from build123d import *

# Parameters (mm, degrees)
SKETCH_1_W           = 200
SKETCH_1_H           = 213
EXTRUDE_1_DEPTH      = 4
EXTRUDE_2_DEPTH      = 54
CUT_EXTRUDE_2_DEPTH  = 298.880848663
CUT_EXTRUDE_3_DEPTH  = 42
SKETCH_7_R           = 1.8
SKETCH_7_R_2         = 11.5
CUT_EXTRUDE_4_DEPTH  = 282.53330176
MIRROR_START         = 176
MIRROR_1_OUTLINE_R   = 1.8
MIRROR_1_OUTLINE_R_2 = 11.5
MIRROR_1_DEPTH       = 3.5
SKETCH_8_W           = 27
SKETCH_8_H           = 28
CUT_EXTRUDE_5_DEPTH  = 6
SKETCH_9_W           = 27
SKETCH_9_H           = 20
CUT_EXTRUDE_6_DEPTH  = 21
CUT_EXTRUDE_START    = -54
CUT_EXTRUDE_7_DEPTH  = 54
SKETCH_12_R          = 2
EXTRUDE_3_DEPTH      = 10
SKETCH_14_W          = 21
SKETCH_14_H          = 20
CUT_EXTRUDE_8_DEPTH  = 297.770955452
SKETCH_15_W          = 6
SKETCH_15_H          = 28
CUT_EXTRUDE_9_DEPTH  = 297.770955452


# Read off the part's stored shape, not the designer's step: 镜向1
with BuildPart() as part:
    # 草图1 → 凸台-拉伸1 (new body)
    with BuildSketch(Plane(origin=(0, 0, 0), x_dir=(1, 0, 0), z_dir=(0, 1, 0))):
        with Locations((100, 106.5)):
            Rectangle(SKETCH_1_W, SKETCH_1_H)
    extrude(amount=EXTRUDE_1_DEPTH)

    # 草图1<4> → 凸台-拉伸2 (add)
    with BuildSketch(Plane(origin=(0, 0, 0), x_dir=(1, 0, 0), z_dir=(0, 1, 0))):
        with BuildLine():
            Line((0, 213), (0, 0))
            ThreePointArc((0, 0), (21.966991411, 53.033008589), (75, 75))
            Line((75, 75), (75, 213))
            Line((75, 213), (0, 213))
        make_face()
        with BuildLine():
            Line((125, 213), (125, 75))
            ThreePointArc((125, 75), (178.033008589, 53.033008589), (200, 0))
            Line((200, 0), (200, 213))
            Line((200, 213), (125, 213))
        make_face()
    extrude(amount=-EXTRUDE_2_DEPTH)

    # 草图3 → 切除-拉伸2 (cut, through all)
    with BuildSketch(Plane.XZ.offset(54)):
        Polygon((20.5, -186), (20.5, -165), (20.5, -144), (20.5, -115), (0, -115), (0, -213), (20.5, -213), align=None)
        Polygon((179.5, -115), (200, -115), (200, -213), (179.5, -213), (179.5, -165), align=None)
    extrude(amount=-CUT_EXTRUDE_2_DEPTH, mode=Mode.SUBTRACT)

    # 草图5 → 切除-拉伸3 (cut)
    with BuildSketch(Plane.XZ.offset(54)):
        Polygon((176, -164), (176, -144), (125, -144), (125, -186), (176, -186), align=None)
        Polygon((24, -164), (24, -144), (75, -144), (75, -186), (24, -186), align=None)
    extrude(amount=-CUT_EXTRUDE_3_DEPTH, mode=Mode.SUBTRACT)

    # 草图7 → 切除-拉伸4 (cut, through all)
    with BuildSketch(Plane(origin=(24, 0, 0), x_dir=(0, 0, -1), z_dir=(1, 0, 0))):
        with Locations((180.5, -17.5)):
            Circle(SKETCH_7_R)
        with Locations((149.5, -17.5)):
            Circle(SKETCH_7_R)
        with Locations((165, -33)):
            Circle(SKETCH_7_R_2)
        with Locations((180.5, -48.5)):
            Circle(SKETCH_7_R)
        with Locations((149.5, -48.5)):
            Circle(SKETCH_7_R)
    extrude(amount=-CUT_EXTRUDE_4_DEPTH, mode=Mode.SUBTRACT)

    # 镜向1 outline → 镜向1 (cut)
    with BuildSketch(Plane.YZ.offset(MIRROR_START)):
        with Locations((-17.5, -180.5)):
            Circle(MIRROR_1_OUTLINE_R)
        with Locations((-17.5, -149.5)):
            Circle(MIRROR_1_OUTLINE_R)
        with Locations((-33, -165)):
            Circle(MIRROR_1_OUTLINE_R_2)
        with Locations((-48.5, -180.5)):
            Circle(MIRROR_1_OUTLINE_R)
        with Locations((-48.5, -149.5)):
            Circle(MIRROR_1_OUTLINE_R)
    extrude(amount=MIRROR_1_DEPTH, mode=Mode.SUBTRACT)

    # 草图8 → 切除-拉伸5 (cut)
    with BuildSketch(Plane(origin=(75, 0, 0), x_dir=(0, 0, -1), z_dir=(1, 0, 0))):
        with Locations((199.5, -33)):
            Rectangle(SKETCH_8_W, SKETCH_8_H)
    extrude(amount=-CUT_EXTRUDE_5_DEPTH, mode=Mode.SUBTRACT)

    # 草图9 → 切除-拉伸6 (cut)
    with BuildSketch(Plane.ZY.offset(-125)):
        with Locations((-199.5, -33)):
            Rectangle(SKETCH_9_W, SKETCH_9_H)
    extrude(amount=-CUT_EXTRUDE_6_DEPTH, mode=Mode.SUBTRACT)

    # 草图11 → 切除-拉伸7 (cut)
    with BuildSketch(Plane.XZ.offset(54).offset(CUT_EXTRUDE_START)):
        with BuildLine():
            Line((29.658534166, -69.684244774), (10.975621098, -39.0625))
            ThreePointArc((10.975621098, -39.0625), (38.289562111, -65.401404801), (75, -75))
            Line((75, -75), (75, -144))
            ThreePointArc((75, -144), (37.483837038, -124.777752739), (31.171635941, -83.099060455))
            ThreePointArc((31.171635941, -83.099060455), (31.899182276, -76.224256342), (29.658534166, -69.684244774))
        make_face()
        with BuildLine():
            Line((125, -144), (125, -75))
            ThreePointArc((125, -75), (161.710437889, -65.401404801), (189.024378902, -39.0625))
            Line((189.024378902, -39.0625), (170.341465834, -69.684244774))
            ThreePointArc((170.341465834, -69.684244774), (168.100817724, -76.224256342), (168.828364059, -83.099060455))
            ThreePointArc((168.828364059, -83.099060455), (162.516162962, -124.777752739), (125, -144))
        make_face()
    extrude(amount=CUT_EXTRUDE_7_DEPTH, mode=Mode.SUBTRACT)

    # 草图12 → 凸台-拉伸3 (add)
    # profile 1 of 2: a face of its own
    with BuildSketch(Plane.XZ.offset(54)):
        with BuildLine():
            Line((18.008349917, -58.289006678), (26.711199556, -66.131863821))
            ThreePointArc((26.711199556, -66.131863821), (32, -78.017578107), (26.711199556, -89.903292393))
            Line((26.711199556, -89.903292393), (18.008349917, -97.746149535))
            ThreePointArc((18.008349917, -97.746149535), (16, -98.517578107), (13.991650083, -97.746149535))
            Line((13.991650083, -97.746149535), (5.288800444, -89.903292393))
            ThreePointArc((5.288800444, -89.903292393), (0, -78.017578107), (5.288800444, -66.131863821))
            Line((5.288800444, -66.131863821), (13.991650083, -58.289006678))
            ThreePointArc((13.991650083, -58.289006678), (16, -57.517578107), (18.008349917, -58.289006678))
        make_face()
        with Locations(Location((16, -60.517578107, 0), (0, 0, 270))):
            Circle(SKETCH_12_R, mode=Mode.SUBTRACT)
        with Locations(Location((16, -95.517578107, 0), (0, 0, 90))):
            Circle(SKETCH_12_R, mode=Mode.SUBTRACT)
    # profile 2 of 2: a face of its own
    with BuildSketch(Plane.XZ.offset(54)):
        with BuildLine():
            Line((186.008349917, -97.746149535), (194.711199556, -89.903292393))
            ThreePointArc((194.711199556, -89.903292393), (200, -78.017578107), (194.711199556, -66.131863821))
            Line((194.711199556, -66.131863821), (186.008349917, -58.289006678))
            ThreePointArc((186.008349917, -58.289006678), (184, -57.517578107), (181.991650083, -58.289006678))
            Line((181.991650083, -58.289006678), (173.288800444, -66.131863821))
            ThreePointArc((173.288800444, -66.131863821), (168, -78.017578107), (173.288800444, -89.903292393))
            Line((173.288800444, -89.903292393), (181.991650083, -97.746149535))
            ThreePointArc((181.991650083, -97.746149535), (184, -98.517578107), (186.008349917, -97.746149535))
        make_face()
        with Locations(Location((184, -95.517578107, 0), (0, 0, 270))):
            Circle(SKETCH_12_R, mode=Mode.SUBTRACT)
        with Locations(Location((184, -60.517578107, 0), (0, 0, 90))):
            Circle(SKETCH_12_R, mode=Mode.SUBTRACT)
    extrude(amount=EXTRUDE_3_DEPTH)

    # 草图14 → 切除-拉伸8 (cut, through all)
    with BuildSketch(Plane.XZ.offset(12)):
        with Locations((64.5, -165)):
            Rectangle(SKETCH_14_W, SKETCH_14_H)
    extrude(amount=-CUT_EXTRUDE_8_DEPTH, mode=Mode.SUBTRACT)

    # 草图15 → 切除-拉伸9 (cut, through all)
    with BuildSketch(Plane.XZ.offset(12)):
        with Locations((128, -165)):
            Rectangle(SKETCH_15_W, SKETCH_15_H)
    extrude(amount=-CUT_EXTRUDE_9_DEPTH, mode=Mode.SUBTRACT)


solid = part.part
Model file for the job. Use its own axes, mm. A direction names the side the tool comes from. Give positions to 0.01 mm unless a question says otherwise; leave off trailing zeros. Loops run counter-clockwise (first coordinate to the right, second up) from the corner with the lowest first, then second, coordinate; pieces in that order, holes last.
Item 1: Drop flat-ended pins along their axis: P1, Ø4, axis at x = 113, z = -84.5, coming from the -Y side; P2, Ø4, axis at y = -10.5, z = -81, coming from the -X side; P3, Ø5, axis at x = 66, y = -6.5, coming from the +Z side; P4, Ø2, axis at y = -17.5, z = -149.5, coming from the -X side. Give the stop position or say it passes through.
Check values:
P1: stops at y = 0
P2: stops at x = 0
P3: stops at z = -142.55
P4: passes through
Item 2: Drill centre lines: line 1 along Y through (x, z) = (177.5, -149.5); line 2 along X through (y, z) = (-47.5, -158.5); line 3 along Z through (x, y) = (176.9, -48.5). Where is each one in solid material? Low to high.
Check values:
line 1: y = -54 to -50.3, -46.7 to -19.3, -15.7 to 4
line 2: x = 20.5 to 24, 176 to 179.5
line 3: z = -213 to -182.3, -178.7 to -151.3, -147.7 to -58.93
Item 3: Slice it at B-B (z = -108). Write the cut outline in (x, y).
Check values:
outline: (0, -54) - (29.92, -54) - (29.92, 0) - (170.08, 0) - (170.08, -54) - (200, -54) - (200, 4) - (0, 4) - close
Item 4: Slice it at A-A (x = 137). Write the cut outline in (y, z), plus the area to 3 significant figures.
Check values:
outline: (-54, -213) - (-43, -213) - (-43, -186) - (-54, -186) - close; (-54, -144) - (-12, -144) - (-12, -186) - (-23, -186) - (-23, -213) - (4, -213) - (4, 0) - (0, 0) - (0, -142.42) - (-54, -142.42) - close
area: 2,360 mm2
Item 5: Which spindle directions (+Z, -Z, +X, -X, +Y, -Y) get a long thin tool onto all of the face, cutting with end or side? Do faces 4 (the face through (75, -6, -149)), 5 (the face through (72, -47, -199)), 6 (the face through (131, -4, -165)), 7 (the face through (176, -24, -156)), 8 (the face through (179.814, -26.622, -54.159)). Say none if no direction does.
Check values:
face 4: +Z, -Z, -Y
face 5: -Z
face 6: +Y, -Y
face 7: -Y
face 8: +Z, -Y
Item 6: Mould opens along X. For faces 1 (the face through (150, -12, -165)), 2 (the face through (16, -64, -78)), 3 (the face through (0, -25, -58)) say: +X half, -X half, draft (parallel to the pull), parting line (faces both ways), or undercut.
Check values:
face 1: undercut
face 2: draft
face 3: -X half
Item 7: Slice it at C-C (x = 35). Write the cut outline in (y, z), plus the area to 3 significant figures.
Check values:
outline: (-54, -213) - (4, -213) - (4, 0) - (0, 0) - (0, -120.94) - (-54, -120.94) - (-54, -144) - (-12, -144) - (-12, -186) - (-54, -186) - close
area: 4,060 mm2
Item 8: Slice it at D-D (z = -73.5). Write the cut outline in (x, y), plus the area to 3 significant figures.
Check values:
outline: (0, -54) - (0.65, -54) - (0.65, -64) - (31.35, -64) - (31.35, 0) - (168.65, 0) - (168.65, -64) - (199.35, -64) - (199.35, -54) - (200, -54) - (200, 4) - (0, 4) - close
area: 4,800 mm2
